```python
from build123d import *

# Parameters (mm, degrees)
BOSS_EXTRUDE1_DEPTH            = 118.4275
CUT_EXTRUDE1_REACH             = 138.757
SKETCH3_R                      = 3.96875
SKETCH3_R_2                    = 3.175
CUT_EXTRUDE1_DIRECTION_2_REACH = 138.757
SKETCH4_R                      = 4.7625
CUT_EXTRUDE2_DEPTH             = 6.35


with BuildPart() as part:
    # Sketch2 → Boss-Extrude1 (new body)
    with BuildSketch(Plane(origin=(0, 0, 0), x_dir=(0, 0, -1), z_dir=(1, 0, 0))):
        Polygon((0, -25.4), (0, 25.4), (-63.5, 25.4), (-63.5, 16.51), (-6.35, 16.51), (-6.35, -16.51), (-63.5, -16.51), (-63.5, -25.4), align=None)
    extrude(amount=BOSS_EXTRUDE1_DEPTH)

    # Cut-Extrude1: up to this face of the body (flat: up to its plane)
    cut_extrude1_end = Plane(part.part.faces().sort_by_distance((59.21375, -25.4, 31.75))[0])
    # Sketch3 → Cut-Extrude1 (cut, up to the picked face)
    with BuildSketch(Plane(origin=(0, 0, 0), x_dir=(1, 0, 0), z_dir=(0, 1, 0)), mode=Mode.PRIVATE) as cut_extrude1_sk1:
        with Locations(Location((7.9375, -19.05, 0), (0, 0, 270))):
            Circle(SKETCH3_R)
    cut_extrude1_tool1 = split(extrude(cut_extrude1_sk1.sketch, amount=-CUT_EXTRUDE1_REACH, mode=Mode.PRIVATE), bisect_by=cut_extrude1_end, keep=Keep.BOTH, mode=Mode.PRIVATE)
    # Sketch3 → Cut-Extrude1 (cut, up to the picked face)
    with BuildSketch(Plane(origin=(0, 0, 0), x_dir=(1, 0, 0), z_dir=(0, 1, 0)), mode=Mode.PRIVATE) as cut_extrude1_sk2:
        with Locations(Location((110.49, -19.05, 0), (0, 0, 270))):
            Circle(SKETCH3_R)
    cut_extrude1_tool2 = split(extrude(cut_extrude1_sk2.sketch, amount=-CUT_EXTRUDE1_REACH, mode=Mode.PRIVATE), bisect_by=cut_extrude1_end, keep=Keep.BOTH, mode=Mode.PRIVATE)
    # Sketch3 → Cut-Extrude1 (cut, up to the picked face)
    with BuildSketch(Plane(origin=(0, 0, 0), x_dir=(1, 0, 0), z_dir=(0, 1, 0)), mode=Mode.PRIVATE) as cut_extrude1_sk3:
        with Locations(Location((40.9575, -13.97, 0), (0, 0, 270))):
            Circle(SKETCH3_R_2)
    cut_extrude1_tool3 = split(extrude(cut_extrude1_sk3.sketch, amount=-CUT_EXTRUDE1_REACH, mode=Mode.PRIVATE), bisect_by=cut_extrude1_end, keep=Keep.BOTH, mode=Mode.PRIVATE)
    # Sketch3 → Cut-Extrude1 (cut, up to the picked face)
    with BuildSketch(Plane(origin=(0, 0, 0), x_dir=(1, 0, 0), z_dir=(0, 1, 0)), mode=Mode.PRIVATE) as cut_extrude1_sk4:
        with BuildLine():
            Line((0, -63.5), (0, -19.05))
            ThreePointArc((0, -19.05), (7.9375, -26.9875), (15.875, -19.05))
            Line((15.875, -19.05), (84.990397552, -19.05))
            ThreePointArc((84.990397552, -19.05), (85.96241347, -18.856654013), (86.786448776, -18.306051224))
            Line((86.786448776, -18.306051224), (92.918551224, -12.173948776))
            ThreePointArc((92.918551224, -12.173948776), (93.74258653, -11.623345987), (94.714602448, -11.43))
            Line((94.714602448, -11.43), (100.0125, -11.43))
            ThreePointArc((100.0125, -11.43), (101.808551224, -12.173948776), (102.5525, -13.97))
            Line((102.5525, -13.97), (102.5525, -19.05))
            ThreePointArc((102.5525, -19.05), (110.49, -26.9875), (118.4275, -19.05))
            Line((118.4275, -19.05), (118.4275, -63.5))
            Line((118.4275, -63.5), (0, -63.5))
        make_face()
    cut_extrude1_tool4 = split(extrude(cut_extrude1_sk4.sketch, amount=-CUT_EXTRUDE1_REACH, mode=Mode.PRIVATE), bisect_by=cut_extrude1_end, keep=Keep.BOTH, mode=Mode.PRIVATE)
    add(cut_extrude1_tool1.solids().sort_by(Axis((7.9375, 0, 19.05), (0, -1, 0)))[0], mode=Mode.SUBTRACT)
    add(cut_extrude1_tool2.solids().sort_by(Axis((110.49, 0, 19.05), (0, -1, 0)))[0], mode=Mode.SUBTRACT)
    add(cut_extrude1_tool3.solids().sort_by(Axis((40.9575, 0, 13.97), (0, -1, 0)))[0], mode=Mode.SUBTRACT)
    add(cut_extrude1_tool4.solids().sort_by(Axis((59.891999, 0, 41.525151), (0, -1, 0)))[0], mode=Mode.SUBTRACT)

    # Cut-Extrude1 direction 2: up to this face of the body (flat: up to its plane)
    cut_extrude1_direction_2_end = Plane(part.part.faces().sort_by_distance((59.21375, 25.4, 31.75))[0])
    # Sketch3 → Cut-Extrude1 direction 2 (cut, up to the picked face)
    with BuildSketch(Plane(origin=(0, 0, 0), x_dir=(1, 0, 0), z_dir=(0, 1, 0)), mode=Mode.PRIVATE) as cut_extrude1_direction_2_sk1:
        with Locations(Location((7.9375, -19.05, 0), (0, 0, 270))):
            Circle(SKETCH3_R)
    cut_extrude1_direction_2_tool1 = split(extrude(cut_extrude1_direction_2_sk1.sketch, amount=CUT_EXTRUDE1_DIRECTION_2_REACH, mode=Mode.PRIVATE), bisect_by=cut_extrude1_direction_2_end, keep=Keep.BOTH, mode=Mode.PRIVATE)
    # Sketch3 → Cut-Extrude1 direction 2 (cut, up to the picked face)
    with BuildSketch(Plane(origin=(0, 0, 0), x_dir=(1, 0, 0), z_dir=(0, 1, 0)), mode=Mode.PRIVATE) as cut_extrude1_direction_2_sk2:
        with Locations(Location((110.49, -19.05, 0), (0, 0, 270))):
            Circle(SKETCH3_R)
    cut_extrude1_direction_2_tool2 = split(extrude(cut_extrude1_direction_2_sk2.sketch, amount=CUT_EXTRUDE1_DIRECTION_2_REACH, mode=Mode.PRIVATE), bisect_by=cut_extrude1_direction_2_end, keep=Keep.BOTH, mode=Mode.PRIVATE)
    # Sketch3 → Cut-Extrude1 direction 2 (cut, up to the picked face)
    with BuildSketch(Plane(origin=(0, 0, 0), x_dir=(1, 0, 0), z_dir=(0, 1, 0)), mode=Mode.PRIVATE) as cut_extrude1_direction_2_sk3:
        with Locations(Location((40.9575, -13.97, 0), (0, 0, 270))):
            Circle(SKETCH3_R_2)
    cut_extrude1_direction_2_tool3 = split(extrude(cut_extrude1_direction_2_sk3.sketch, amount=CUT_EXTRUDE1_DIRECTION_2_REACH, mode=Mode.PRIVATE), bisect_by=cut_extrude1_direction_2_end, keep=Keep.BOTH, mode=Mode.PRIVATE)
    # Sketch3 → Cut-Extrude1 direction 2 (cut, up to the picked face)
    with BuildSketch(Plane(origin=(0, 0, 0), x_dir=(1, 0, 0), z_dir=(0, 1, 0)), mode=Mode.PRIVATE) as cut_extrude1_direction_2_sk4:
        with BuildLine():
            Line((0, -63.5), (0, -19.05))
            ThreePointArc((0, -19.05), (7.9375, -26.9875), (15.875, -19.05))
            Line((15.875, -19.05), (84.990397552, -19.05))
            ThreePointArc((84.990397552, -19.05), (85.96241347, -18.856654013), (86.786448776, -18.306051224))
            Line((86.786448776, -18.306051224), (92.918551224, -12.173948776))
            ThreePointArc((92.918551224, -12.173948776), (93.74258653, -11.623345987), (94.714602448, -11.43))
            Line((94.714602448, -11.43), (100.0125, -11.43))
            ThreePointArc((100.0125, -11.43), (101.808551224, -12.173948776), (102.5525, -13.97))
            Line((102.5525, -13.97), (102.5525, -19.05))
            ThreePointArc((102.5525, -19.05), (110.49, -26.9875), (118.4275, -19.05))
            Line((118.4275, -19.05), (118.4275, -63.5))
            Line((118.4275, -63.5), (0, -63.5))
        make_face()
    cut_extrude1_direction_2_tool4 = split(extrude(cut_extrude1_direction_2_sk4.sketch, amount=CUT_EXTRUDE1_DIRECTION_2_REACH, mode=Mode.PRIVATE), bisect_by=cut_extrude1_direction_2_end, keep=Keep.BOTH, mode=Mode.PRIVATE)
    add(cut_extrude1_direction_2_tool1.solids().sort_by(Axis((7.9375, 0, 19.05), (0, 1, 0)))[0], mode=Mode.SUBTRACT)
    add(cut_extrude1_direction_2_tool2.solids().sort_by(Axis((110.49, 0, 19.05), (0, 1, 0)))[0], mode=Mode.SUBTRACT)
    add(cut_extrude1_direction_2_tool3.solids().sort_by(Axis((40.9575, 0, 13.97), (0, 1, 0)))[0], mode=Mode.SUBTRACT)
    add(cut_extrude1_direction_2_tool4.solids().sort_by(Axis((59.891999, 0, 41.525151), (0, 1, 0)))[0], mode=Mode.SUBTRACT)

    # Sketch4 → Cut-Extrude2 (cut)
    with BuildSketch(Plane.XY):
        with Locations(Location((19.05, 0, 0), (0, 0, 180))):
            Circle(SKETCH4_R)
        with Locations(Location((99.3775, 0, 0), (0, 0, 180))):
            Circle(SKETCH4_R)
    extrude(amount=CUT_EXTRUDE2_DEPTH, mode=Mode.SUBTRACT)


solid = part.part
```
Model file for the job. Use its own axes, mm. A direction names the side the tool comes from. Coordinates: 2 decimals unless noted, no trailing zeros. Order: outer loops, then holes, each group sorted by start corner. A loop starts at its lowest first (then second) coordinate and runs counter-clockwise, first axis right, second up. Notation, with made-up numbers: (-22.5, 1.5) -> (36.5, 1.5) arc R16 ccw to (36.5, 11.5) -> close; hole circle Ø10 at (38, 75.25). An arc over 180 degrees is marked (long way). Answer as a JSON object with one key per item and string values. Group by question number.
1) Flat gauge pins, fed straight in: pin 1 (2.5 mm diameter, centred on x = 49.5, y = 19.5, fed in from +Z); pin 2 (4 mm diameter, centred on x = 97.5, y = 19, fed in from +Z); pin 3 (11 mm diameter, centred on x = 99.38, y = 0, fed in from +Z); pin 4 (7 mm diameter, centred on x = 7.94, z = 19.05, fed in from +Y). Where does each tip first touch, or does it go through?
2) Cut at D-D, the plane x = 26.5. Write the cut outline in (y, z), then the cut area to 3 significant figures.
3) Cut at B-B, the plane x = 110.49. Write the cut outline in (y, z), then the cut area to 3 significant figures.
4) Drill centre lines: L1, parallel to Y at x = 19.05, z = 5.25; L2, parallel to X at y = -21, z = 13.97; L3, parallel to Y at x = 100, z = 8.75. Where is each one in solid material? Low to high.
5) Pull direction Y, two halves, no side cores. Call faces 1 (the face through (58, 25.4, 10)), 2 (the face through (101.789, -20.893, 12.154)), 3 (the face through (104.135, -0.209, 3.131)): +Y half, -Y half, draft (parallel to the pull), parting line (faces both ways), or undercut.
6) Cut at C-C, the plane z = 9.25. Write the cut outline in (x, y).
7) Which spindle directions (+Z, -Z, +X, -X, +Y, -Y) get a long thin tool onto all of the face, cutting with end or side? Do faces 4 (the face through (101.789, 20.893, 12.154)), 5 (the face through (58, 16.51, 12)), 6 (the face through (106.616, 20.893, 18.19)). Say none if no direction does.
8) Cut at A-A, the plane y = 0. Count the separate pieces of the cut face and the enclosed holes in it, then the cut area to 3 significant figures.
Check values:
{
 "1": {"pin 1": "stops at z = 19.05", "pin 2": "stops at z = 11.43", "pin 3": "stops at z = 6.35", "pin 4": "passes through"},
 "2": {"outline": "(-25.4, 0) -> (25.4, 0) -> (25.4, 19.05) -> (16.51, 19.05) -> (16.51, 6.35) -> (-16.51, 6.35) -> (-16.51, 19.05) -> (-25.4, 19.05) -> close", "area": "548 mm²"},
 "3": {"outline": "(-25.4, 0) -> (25.4, 0) -> (25.4, 15.08) -> (16.51, 15.08) -> (16.51, 6.35) -> (-16.51, 6.35) -> (-16.51, 15.08) -> (-25.4, 15.08) -> close; (-25.4, 23.02) -> (-16.51, 23.02) -> (-16.51, 26.99) -> (-25.4, 26.99) -> close; (16.51, 23.02) -> (25.4, 23.02) -> (25.4, 26.99) -> (16.51, 26.99) -> close", "area": "548 mm²"},
 "4": {"L1": "y = -25.4 to -4.76, 4.76 to 25.4", "L2": "x = 0 to 37.78, 44.13 to 91.12, 102.55 to 118.43", "L3": "y = -25.4 to -16.51, 16.51 to 25.4"},
 "5": {"face 1": "+Y half", "face 2": "draft", "face 3": "undercut"},
 "6": {"outline": "(0, -25.4) -> (118.43, -25.4) -> (118.43, -16.51) -> (0, -16.51) -> close; (0, 16.51) -> (118.43, 16.51) -> (118.43, 25.4) -> (0, 25.4) -> close"},
 "7": {"face 4": "+Z, +Y, -Y", "face 5": "+Z, +X, -X", "face 6": "+Y, -Y"},
 "8": {"separate pieces": "3", "enclosed holes": "0", "area": "631 mm²"}
}
